Can you work these out from the model? Positions are in its coordinate system, mm. Face numbers are marked on the shaded views. A direction names the side the tool comes from. Give positions to 0.01 mm unless a question says otherwise; leave off trailing zeros. Order: outer loops, then holes, each group sorted by start corner. A loop starts at its lowest first (then second) coordinate and runs counter-clockwise, first axis right, second up. Notation, with made-up numbers: M 76,23.5 L 114,23.5 A11 ccw 114,34.5 Z; hole C -18,84 d7. An arc over 180 degrees is marked long. Answer as a JSON object with one key per item and string values.
```python
from build123d import *

# Parameters (mm, degrees)
SKETCH_1_W          = 40.4
SKETCH_1_H          = 19.8
EXTRUDE_1_DEPTH     = 2
SKETCH_2_W          = 38.4
SKETCH_2_H          = 17.9
EXTRUDE_2_DEPTH     = 2
CUT_EXTRUDE_6_DEPTH = 1
EXTRUDE_7_DEPTH     = 0.7
SKETCH_4_R          = 0.8
CUT_EXTRUDE_4_DEPTH = 23.848413512
SKETCH_8_W          = 2
SKETCH_8_H          = 5
CUT_EXTRUDE_8_DEPTH = 1.8


with BuildPart() as part:
    # 草圖1 → 伸長1 (new body)
    with BuildSketch(Plane.XY):
        Rectangle(SKETCH_1_W, SKETCH_1_H)
    extrude(amount=EXTRUDE_1_DEPTH)

    # 草圖2 → 伸長2 (add)
    with BuildSketch(Plane(origin=(0, 0, 0), x_dir=(-1, 0, 0), z_dir=(0, 0, 1))):
        Rectangle(SKETCH_2_W, SKETCH_2_H)
        with BuildLine():
            Line((-15.485164876, 8.15), (15.485164876, 8.15))
            ThreePointArc((15.485164876, 8.15), (16.512994231, 6.262994231), (18.4, 5.235164876))
            Line((18.4, 5.235164876), (18.4, -5.235164876))
            ThreePointArc((18.4, -5.235164876), (16.512994231, -6.262994231), (15.485164876, -8.15))
            Line((15.485164876, -8.15), (-15.485164876, -8.15))
            ThreePointArc((-15.485164876, -8.15), (-16.512994231, -6.262994231), (-18.4, -5.235164876))
            Line((-18.4, -5.235164876), (-18.4, 5.235164876))
            ThreePointArc((-18.4, 5.235164876), (-16.512994231, 6.262994231), (-15.485164876, 8.15))
        make_face(mode=Mode.SUBTRACT)
    extrude(amount=-EXTRUDE_2_DEPTH)

    # 草圖5 → 伸長6 (cut)
    with BuildSketch(Plane.XY.offset(2)):
        with BuildLine():
            Line((14.771682035, 8.15), (14.771682035, 9.9))
            Line((14.771682035, 9.9), (20.2, 9.9))
            Line((20.2, 9.9), (20.2, 4.521682035))
            Line((20.2, 4.521682035), (18.4, 4.521682035))
            ThreePointArc((18.4, 4.521682035), (16.018019485, 5.768019485), (14.771682035, 8.15))
        make_face()
        with BuildLine():
            Line((-14.771682035, 8.15), (-14.771682035, 9.9))
            Line((-14.771682035, 9.9), (-20.2, 9.9))
            Line((-20.2, 9.9), (-20.2, 4.521682035))
            Line((-20.2, 4.521682035), (-18.4, 4.521682035))
            ThreePointArc((-18.4, 4.521682035), (-16.018019485, 5.768019485), (-14.771682035, 8.15))
        make_face()
        with BuildLine():
            Line((-18.4, -4.521682035), (-20.2, -4.521682035))
            Line((-20.2, -4.521682035), (-20.2, -9.9))
            Line((-20.2, -9.9), (-14.771682035, -9.9))
            Line((-14.771682035, -9.9), (-14.771682035, -8.15))
            ThreePointArc((-14.771682035, -8.15), (-16.018019485, -5.768019485), (-18.4, -4.521682035))
        make_face()
        with BuildLine():
            Line((14.771682035, -8.15), (14.771682035, -9.9))
            Line((14.771682035, -9.9), (20.2, -9.9))
            Line((20.2, -9.9), (20.2, -4.521682035))
            Line((20.2, -4.521682035), (18.4, -4.521682035))
            ThreePointArc((18.4, -4.521682035), (16.018019485, -5.768019485), (14.771682035, -8.15))
        make_face()
    extrude(amount=-CUT_EXTRUDE_6_DEPTH, mode=Mode.SUBTRACT)

    # 草圖6 → 伸長7 (add)
    with BuildSketch(Plane(origin=(0, 0, 0), x_dir=(-1, 0, 0), z_dir=(0, 0, -1))):
        with BuildLine():
            Line((-19.2, -4.45), (-19.2, -8.95))
            Line((-19.2, -8.95), (-14.7, -8.95))
            ThreePointArc((-14.7, -8.95), (-16.018019485, -5.768019485), (-19.2, -4.45))
        make_face()
        with BuildLine():
            Line((-19.2, 8.95), (-14.7, 8.95))
            ThreePointArc((-14.7, 8.95), (-16.018019485, 5.768019485), (-19.2, 4.45))
            Line((-19.2, 4.45), (-19.2, 8.95))
        make_face()
        with BuildLine():
            Line((19.2, 8.95), (19.2, 4.45))
            ThreePointArc((19.2, 4.45), (16.018019485, 5.768019485), (14.7, 8.95))
            Line((14.7, 8.95), (19.2, 8.95))
        make_face()
        with BuildLine():
            Line((14.7, -8.95), (19.2, -8.95))
            Line((19.2, -8.95), (19.2, -4.45))
            ThreePointArc((19.2, -4.45), (16.018019485, -5.768019485), (14.7, -8.95))
        make_face()
    extrude(amount=EXTRUDE_7_DEPTH)

    # 草圖4 → 伸長4 (cut, through all)
    with BuildSketch(Plane(origin=(0, 0, 2), x_dir=(-1, 0, 0), z_dir=(0, 0, 1))):
        with Locations(Location((-17.7, 7.4, 0), (0, 0, 180))):
            Circle(SKETCH_4_R)
        with Locations(Location((17.7, 7.4, 0), (0, 0, 180))):
            Circle(SKETCH_4_R)
        with Locations(Location((17.7, -7.4, 0), (0, 0, 180))):
            Circle(SKETCH_4_R)
        with Locations(Location((-17.7, -7.4, 0), (0, 0, 180))):
            Circle(SKETCH_4_R)
    extrude(amount=-CUT_EXTRUDE_4_DEPTH, mode=Mode.SUBTRACT)

    # 草圖8 → 伸長8 (cut)
    with BuildSketch(Plane(origin=(20.2, 0, 0), x_dir=(0, 0, -1), z_dir=(1, 0, 0))):
        with Locations((1, 0)):
            Rectangle(SKETCH_8_W, SKETCH_8_H)
    extrude(amount=-CUT_EXTRUDE_8_DEPTH, mode=Mode.SUBTRACT)


solid = part.part
```
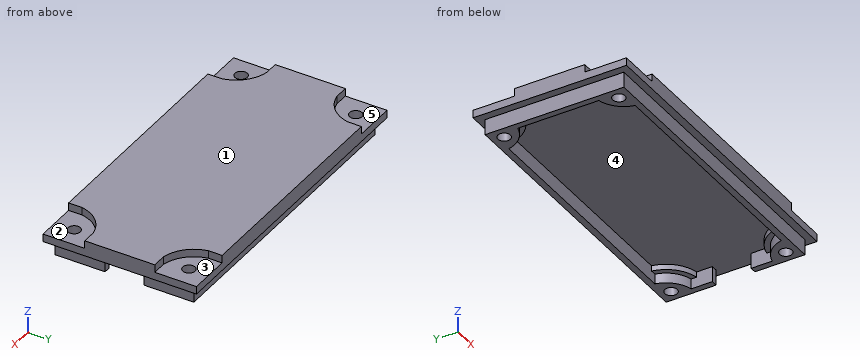
1) I want a section at D-D on y = -7.4. Write out the boundary of the cut face in (x, z).
Results found:
{"outline": "M -20.2,0 L -19.2,0 L -19.2,-2 L -18.5,-2 L -18.5,1 L -20.2,1 Z; M -16.9,-2 L -15.73,-2 L -15.73,-0.7 L -14.98,-0.7 L -14.98,0 L 14.98,0 L 14.98,-0.7 L 15.73,-0.7 L 15.73,-2 L 16.9,-2 L 16.9,1 L 14.98,1 L 14.98,2 L -14.98,2 L -14.98,1 L -16.9,1 Z; M 18.5,-2 L 19.2,-2 L 19.2,0 L 20.2,0 L 20.2,1 L 18.5,1 Z"}
2) I want a section at B-B on y = -3.25. Write out the boundary of the cut face in (x, z), and give its area (3 significant figures).
Results found:
{"outline": "M -20.2,0 L -19.2,0 L -19.2,-2 L -18.4,-2 L -18.4,0 L 18.4,0 L 18.4,-2 L 19.2,-2 L 19.2,0 L 20.2,0 L 20.2,2 L -20.2,2 Z", "area": "84.0 mm²"}
3) I need wall thicknesses on L1, parallel to X at y = 7.5, z = 0.05; L2, parallel to Y at x = 17, z = 0.55; L3, parallel to Y at x = -18, z = 0.5. Which ranges of each line are inside material? Lowest first, please.
Results found:
{"L1": "x = -20.2 to -18.49, -16.91 to 16.91, 18.49 to 20.2", "L2": "y = -9.9 to -7.79, -7.01 to 7.01, 7.79 to 9.9", "L3": "y = -9.9 to -8.14, -6.66 to 6.66, 8.14 to 9.9"}
4) Thinking about a two-plate mould opening in Y: for the marked faces 4 and 5, which applies, pulls with the +Y half, pulls with the -Y half, needs draft (parallel to the pull), parting line crosses it, or undercut?
Results found:
{"face 4": "undercut", "face 5": "needs draft"}
5) I want a section at A-A on z = -1.6. Write out the boundary of the cut face in (x, y).
Results found:
{"outline": "M -19.2,-8.95 L 19.2,-8.95 L 19.2,-2.5 L 18.4,-2.5 L 18.4,-5.24 A3.8 ccw 15.49,-8.15 L -15.49,-8.15 A3.8 ccw -18.4,-5.24 L -18.4,5.24 A3.8 ccw -15.49,8.15 L 15.49,8.15 A3.8 ccw 18.4,5.24 L 18.4,2.5 L 19.2,2.5 L 19.2,8.95 L -19.2,8.95 Z; hole C -17.7,-7.4 d1.6; hole C -17.7,7.4 d1.6; hole C 17.7,-7.4 d1.6; hole C 17.7,7.4 d1.6"}
6) I want a section at C-C on x = 17.7. Write out the boundary of the cut face in (y, z), and give its area (3 significant figures).
Results found:
{"outline": "M -9.9,0 L -8.95,0 L -8.95,-2 L -8.2,-2 L -8.2,1 L -9.9,1 Z; M -6.6,-2 L -5.46,-2 L -5.46,-0.7 L -4.71,-0.7 L -4.71,0 L 4.71,0 L 4.71,-0.7 L 5.46,-0.7 L 5.46,-2 L 6.6,-2 L 6.6,1 L 4.71,1 L 4.71,2 L -4.71,2 L -4.71,1 L -6.6,1 Z; M 8.2,-2 L 8.95,-2 L 8.95,0 L 9.9,0 L 9.9,1 L 8.2,1 Z", "area": "34.6 mm²"}
7) I'm going to push flat-ended pins straight in: pin 1 Ø2 at (x, z) = (2, -1.5) entering from +Y; pin 2 Ø0.5 at (x, z) = (19.5, 1.5) entering from +Y; pin 3 Ø6 at (x, y) = (14.5, -0.5) entering from -Z. Where does each tip first touch, or does it pass through?
Results found:
{"pin 1": "stops at y = 8.95", "pin 2": "stops at y = 4.52", "pin 3": "stops at z = 0"}
8) For the marked faces 1, 2 and 3, which set-ups out of +Z, -Z, +X, -X, +Y, -Y let a thin tool reach every point of the face, with its end or its side?
Results found:
{"face 1": "+Z, +X, -X, +Y, -Y", "face 2": "+Z, +X, -Y", "face 3": "+Z, +X, +Y"}
